from build123d import *

# Parameters (mm, degrees)
SKETCH1_W           = 76.8
SKETCH1_H           = 61.3
BOSS_EXTRUDE1_DEPTH = 2
SKETCH2_W           = 76.8
SKETCH2_H           = 61.3
SKETCH2_W_2         = 70.8
SKETCH2_H_2         = 55.3
BOSS_EXTRUDE2_DEPTH = 15
CUT_EXTRUDE1_REACH  = 86.04
SKETCH6_W           = 13
SKETCH6_H           = 14.670742809
CUT_EXTRUDE2_REACH  = 86.04
SKETCH7_W           = 9.9
SKETCH7_H           = 11.743698963
CUT_EXTRUDE3_REACH  = 75.873
SKETCH8_W           = 41
SKETCH8_H           = 11.477298103
CUT_EXTRUDE4_REACH  = 75.873
SKETCH9_W           = 50
SKETCH9_H           = 13.6396876
SKETCH10_R          = 1.75
BOSS_EXTRUDE4_DEPTH = 2
SKETCH11_R          = 0.75
CUT_EXTRUDE5_DEPTH  = 2.5
SKETCH12_R          = 0.75
CUT_EXTRUDE6_DEPTH  = 2.5


with BuildPart() as part:
    # Sketch1 → Boss-Extrude1 (new body)
    with BuildSketch(Plane(origin=(0, 0, 0), x_dir=(1, 0, 0), z_dir=(0, 1, 0))):
        Rectangle(SKETCH1_W, SKETCH1_H)
    extrude(amount=-BOSS_EXTRUDE1_DEPTH)

    # Sketch2 → Boss-Extrude2 (add)
    with BuildSketch(Plane(origin=(0, 0, 0), x_dir=(1, 0, 0), z_dir=(0, 1, 0))):
        Rectangle(SKETCH2_W, SKETCH2_H)
        Rectangle(SKETCH2_W_2, SKETCH2_H_2, mode=Mode.SUBTRACT)
    extrude(amount=BOSS_EXTRUDE2_DEPTH)

    # Sketch6 → Cut-Extrude1 (cut, up to next)
    with BuildSketch(Plane.ZY.offset(38.4), mode=Mode.PRIVATE) as cut_extrude1_sk1:
        with Locations((-12.05, 10.935371405)):
            Rectangle(SKETCH6_W, SKETCH6_H)
    cut_extrude1_tool1 = extrude(cut_extrude1_sk1.sketch, amount=-CUT_EXTRUDE1_REACH, mode=Mode.PRIVATE) & part.part
    add(cut_extrude1_tool1.solids().sort_by_distance((-38.4, 10.935371, -12.05))[0], mode=Mode.SUBTRACT)

    # Sketch7 → Cut-Extrude2 (cut, up to next)
    with BuildSketch(Plane.ZY.offset(38.4), mode=Mode.PRIVATE) as cut_extrude2_sk1:
        with Locations((19.9, 9.471849482)):
            Rectangle(SKETCH7_W, SKETCH7_H)
    cut_extrude2_tool1 = extrude(cut_extrude2_sk1.sketch, amount=-CUT_EXTRUDE2_REACH, mode=Mode.PRIVATE) & part.part
    add(cut_extrude2_tool1.solids().sort_by_distance((-38.4, 9.471849, 19.9))[0], mode=Mode.SUBTRACT)

    # Sketch8 → Cut-Extrude3 (cut, up to next)
    with BuildSketch(Plane.XY.offset(30.65), mode=Mode.PRIVATE) as cut_extrude3_sk1:
        with Locations((11.9, 17.738649052)):
            Rectangle(SKETCH8_W, SKETCH8_H)
    cut_extrude3_tool1 = extrude(cut_extrude3_sk1.sketch, amount=-CUT_EXTRUDE3_REACH, mode=Mode.PRIVATE) & part.part
    add(cut_extrude3_tool1.solids().sort_by_distance((11.9, 17.738649, 30.65))[0], mode=Mode.SUBTRACT)

    # Sketch9 → Cut-Extrude4 (cut, up to next)
    with BuildSketch(Plane(origin=(0, 0, -30.65), x_dir=(-1, 0, 0), z_dir=(0, 0, -1)), mode=Mode.PRIVATE) as cut_extrude4_sk1:
        with Locations((-7.4, 18.8198438)):
            Rectangle(SKETCH9_W, SKETCH9_H)
    cut_extrude4_tool1 = extrude(cut_extrude4_sk1.sketch, amount=-CUT_EXTRUDE4_REACH, mode=Mode.PRIVATE) & part.part
    add(cut_extrude4_tool1.solids().sort_by_distance((7.4, 18.819844, -30.65))[0], mode=Mode.SUBTRACT)

    # Sketch10 → Boss-Extrude4 (add)
    with BuildSketch(Plane(origin=(0, 0, 0), x_dir=(1, 0, 0), z_dir=(0, 1, 0))):
        with Locations(Location((-19.3, 23.65, 0), (0, 0, 90))):
            Circle(SKETCH10_R)
        with Locations(Location((-20.4, -24.15, 0), (0, 0, 90))):
            Circle(SKETCH10_R)
        with Locations(Location((31.5, 8.45, 0), (0, 0, 90))):
            Circle(SKETCH10_R)
        with Locations(Location((31.5, -19.45, 0), (0, 0, 90))):
            Circle(SKETCH10_R)
    extrude(amount=BOSS_EXTRUDE4_DEPTH)

    # Sketch11 → Cut-Extrude5 (cut)
    with BuildSketch(Plane(origin=(0, 2, 0), x_dir=(1, 0, 0), z_dir=(0, 1, 0))):
        with Locations(Location((-19.3, 23.65, 0), (0, 0, 270))):
            Circle(SKETCH11_R)
        with Locations(Location((-20.4, -24.15, 0), (0, 0, 270))):
            Circle(SKETCH11_R)
        with Locations(Location((31.5, 8.45, 0), (0, 0, 270))):
            Circle(SKETCH11_R)
        with Locations(Location((31.5, -19.45, 0), (0, 0, 270))):
            Circle(SKETCH11_R)
    extrude(amount=-CUT_EXTRUDE5_DEPTH, mode=Mode.SUBTRACT)

    # Sketch12 → Cut-Extrude6 (cut)
    with BuildSketch(Plane(origin=(0, 15, 0), x_dir=(1, 0, 0), z_dir=(0, 1, 0))):
        with Locations(Location((-37, 29, 0), (0, 0, 270))):
            Circle(SKETCH12_R)
        with Locations(Location((37, 29, 0), (0, 0, 270))):
            Circle(SKETCH12_R)
        with Locations(Location((37, -29, 0), (0, 0, 270))):
            Circle(SKETCH12_R)
        with Locations(Location((-37, -29, 0), (0, 0, 270))):
            Circle(SKETCH12_R)
    extrude(amount=-CUT_EXTRUDE6_DEPTH, mode=Mode.SUBTRACT)


solid = part.part
For this review, take the finished solid that the model builds, in its own axes (mm). A direction names the side the tool comes from. Give positions to 0.01 mm unless a question says otherwise; leave off trailing zeros. Loops run counter-clockwise (first coordinate to the right, second up) from the corner with the lowest first, then second, coordinate; pieces in that order, holes last. Notation, with made-up numbers: M -20,-2.75 L 37,-2.75 A13 ccw 37,12.25 Z; hole C -33,-21 d5. An arc over 180 degrees is marked long. Answer as a JSON object with one key per item and string values. Group by question number.
Q1. Add section C-C on z = 13.5. Give the boundary of the cut face in (x, y).
Q2. Tool access review of faces 4 (the cylindrical face through (-18.85, 0.99, 23.34)), 5 (the flat face through (32.4, 13, 29)), 6 (the flat face through (8, 12, -29)): name each direction out of +Z, -Z, +X, -X, +Y, -Y from which nothing blocks a thin tool from reaching the whole face with its end or side.
Q3. Insertion check: P1, Ø3.5, axis at x = 20, z = -29, coming from the +Y side; P2, Ø1, axis at x = 18, z = -8, coming from the +Y side; P3, Ø0.8, axis at x = 37, z = -29, coming from the +Y side. Each pin has a flat end and moves straight along its axis. Give the tip position at first contact, or say it passes through.
Q4. Mouldability with a two-part tool opening along Z and no side actions: class faces 1 (the flat face through (35.4, 7, 0)), 2 (the flat face through (12, 12, 29)), 3 (the flat face through (-1, 6, 30.65)) as +Z half, -Z half, draft (parallel to the pull), parting line (faces both ways), or undercut.
Q5. For probe 1 along Z at (x, y) = (37, 13.9); probe 2 along X at (y, z) = (14.2, -29); probe 3 along X at (y, z) = (0.5, -8.45), list the stretches that pass through material, from the lowest coordinate up. Write a range as [from, to].
Q6. Add section B-B on x = 8. Give the boundary of the cut face in (y, z).
Q7. Add section A-A on y = 10.75. Give the boundary of the cut face in (x, z), and give its area (3 significant figures).
Checked values:
{
 "1": {"outline": "M -38.4,-2 L 38.4,-2 L 38.4,15 L 35.4,15 L 35.4,0 L -35.4,0 L -35.4,15 L -38.4,15 Z"},
 "2": {"face 4": "+Y", "face 5": "+Z, -Z, +Y", "face 6": "-Z, +Y"},
 "3": {"P1": "y = 12", "P2": "y = 0", "P3": "y = 12.5"},
 "4": {"face 1": "undercut", "face 2": "draft", "face 3": "+Z half"},
 "5": {"probe 1": "[-30.65, -29.75], [-28.25, 28.25], [29.75, 30.65]", "probe 2": "[-38.4, -37.75], [-36.25, -17.6], [32.4, 36.25], [37.75, 38.4]", "probe 3": "[-38.4, -35.4], [29.75, 30.75], [32.25, 33.25], [35.4, 38.4]"},
 "6": {"outline": "M -2,-30.65 L 12,-30.65 L 12,-27.65 L 0,-27.65 L 0,27.65 L 12,27.65 L 12,30.65 L -2,30.65 Z"},
 "7": {"outline": "M -38.4,-30.65 L 38.4,-30.65 L 38.4,30.65 L -38.4,30.65 L -38.4,24.85 L -35.4,24.85 L -35.4,27.65 L 35.4,27.65 L 35.4,-27.65 L -35.4,-27.65 L -35.4,-18.55 L -38.4,-18.55 Z; M -38.4,-5.55 L -35.4,-5.55 L -35.4,14.95 L -38.4,14.95 Z", "area": "724 mm²"}
}
